Read the model definition and answer for the solid it produces. Units are mm, in the model's axes. A direction names the side the tool comes from. Coordinates: 2 decimals unless noted, no trailing zeros. Order: outer loops, then holes, each group sorted by start corner. A loop starts at its lowest first (then second) coordinate and runs counter-clockwise, first axis right, second up. Notation, with made-up numbers: (-37, -1.75) - (4, -1.75) arc R28 ccw to (4, 21.25) - close; hole circle Ø11 at (-27.75, -16.75). An arc over 180 degrees is marked (long way). Answer as a JSON object with one key per item and string values. Group by question number.
from build123d import *

# Parameters (mm, degrees)
F0_W     = 75.8960098028
F0_H     = 49.6515966952
F1_DEPTH = 50.8
F3_DEPTH = 25.4
F4_R     = 17.7026194938
F5_DEPTH = 50.8


with BuildPart() as f1:
    # F0 (on Front) → F1 (new body)
    with BuildSketch(Plane.XZ):
        with Locations((37.9480049014, 24.8257983476)):
            Rectangle(F0_W, F0_H)
    extrude(amount=F1_DEPTH)

    # F2 (on face) → F3 (cut)
    with BuildSketch(Plane.XZ.offset(50.8)):
        Polygon((75.8960098028, 49.6515966952), (23.1234580278, 49.6515966952), (50.928350538, 0), (75.8960098028, 0), align=None)
    extrude(amount=-F3_DEPTH, mode=Mode.SUBTRACT)

    # F4 (on face) → F5 (cut)
    with BuildSketch(Plane.XZ.offset(50.8)):
        with Locations((31.635157764, 21.5629786253)):
            Circle(F4_R)
    extrude(amount=-F5_DEPTH, mode=Mode.SUBTRACT)


solid = f1.part
1. A cutting plane is placed at B-B on z = 36.5. Write down the section's boundary in (x, y), and give its area (3 significant figures).
2. For faces 1 (the flat face through (55, -25.4, 31)), 2 (the flat face through (0, -25, 24)), determine the directions among +Z, -Z, +X, -X, +Y, -Y from which every point of the face is accessible in a straight line to the end or side of a thin tool.
3. Straight lines are drawn through the part: L1, parallel to X at y = -9, z = 25.5; L2, parallel to Y at x = 30, z = 41; L3, parallel to Z at x = 48, y = -13.5. For each, find the intervals that lie inside material, in ascending order.
4. A cutting plane is placed at A-A on x = 20.5. Write down the section's boundary in (y, z).
5. A cutting plane is placed at C-C on y = -47. Write down the section's boundary in (x, z).
6. For a pull along Z with two mould halves and no side action, classify faces 3 (the cylindrical face through (17.59, -20.11, 10.79)), 4 (the flat face through (46, 0, 36)), 5 (the flat face through (29, -19, 49.652)) as pulls with the +Z half, pulls with the -Z half, needs draft (parallel to the pull), parting line crosses it, or undercut.
7. A cutting plane is placed at D-D on y = -15. Write down the section's boundary in (x, z).
8. Given pin 1 (12 mm diameter, centred on y = -35.5, z = 12, fed in from +X); pin 2 (15 mm diameter, centred on x = 53.5, z = 20.5, fed in from -Y), each flat-ended and moving along its own axis, determine where each tip first touches the part or whether it passes through.
Derived:
{
 "1": {"outline": "(0, -50.8) - (22.13, -50.8) - (22.13, 0) - (0, 0) - close; (41.14, -25.4) - (75.9, -25.4) - (75.9, 0) - (41.14, 0) - close", "area": "2,010 mm2"},
 "2": {"face 1": "+Z, +X, -Y", "face 2": "+Z, -Z, -X, +Y, -Y"},
 "3": {"L1": "x = 0 to 14.38, 48.89 to 75.9", "L2": "y = -25.4 to 0", "L3": "z = 0 to 14.81, 28.31 to 49.65"},
 "4": {"outline": "(-50.8, 0) - (0, 0) - (0, 7.8) - (-50.8, 7.8) - close; (-50.8, 35.32) - (0, 35.32) - (0, 49.65) - (-50.8, 49.65) - close"},
 "5": {"outline": "(0, 0) - (50.93, 0) - (45.21, 10.2) arc R17.7 cw (long way) to (29.05, 39.08) - (23.12, 49.65) - (0, 49.65) - close"},
 "6": {"face 3": "undercut", "face 4": "needs draft", "face 5": "pulls with the +Z half"},
 "7": {"outline": "(0, 0) - (75.9, 0) - (75.9, 49.65) - (0, 49.65) - close; hole circle Ø35.41 at (31.64, 21.56)"},
 "8": {"pin 1": "stops at x = 47.57", "pin 2": "stops at y = -25.4"}
}
